Design review of the part built by this model. Coordinates are the model's own, in mm. A direction names the side the tool comes from. Give positions to 0.01 mm unless a question says otherwise; leave off trailing zeros. Loops run counter-clockwise (first coordinate to the right, second up) from the corner with the lowest first, then second, coordinate; pieces in that order, holes last. Notation, with made-up numbers: (0, -11) - (43, -11) arc R30 ccw to (43, 26) - close; hole circle Ø1 at (-15, 11). An arc over 180 degrees is marked (long way). Write each question's results on one line, items separated by ' | '.
```python
from build123d import *

# Parameters (mm, degrees)
F2_SIZE = 1


with BuildPart() as f1:
    # F0 (on Front) → F1 (revolve)
    with BuildSketch(Plane.XZ):
        Polygon((-27.5, 0), (-22, 0), (-22, 13), (-19, 13), (-19, 25), (-22, 25), (-22, 38), (-27.5, 38), (-27.5, 36), (-26, 36), (-26, 27), (-27.5, 27), (-27.5, 11), (-26, 11), (-26, 2), (-27.5, 2), align=None)
    revolve(axis=Axis((0, 0, 48.059855), (0, 0, 1)))

    # F2
    f2_edges = [f1.edges().sort_by_distance(p)[0] for p in [
        (22, 0, 38),
        (22, 0, 0),
    ]]
    chamfer(f2_edges, length=F2_SIZE)


solid = f1.part
```
Item 1: Tool access review of faces 1 (the face through (-7, -18, 25)), 2 (the face through (20.633, 15.821, 6.437)), 3 (the face through (-14.4, 18.2, 38)), 4 (the face through (7, -18, 13)): name each direction out of +Z, -Z, +X, -X, +Y, -Y from which nothing blocks a thin tool from reaching the whole face with its end or side.
Output values:
face 1: +Z | face 2: none | face 3: +Z, +X, -X, +Y, -Y | face 4: -Z
Item 2: Wall thickness on probe 1 along Z at (x, y) = (-20, -17); probe 2 along Y at (x, z) = (0, 5.5); probe 3 along Y at (x, z) = (0, 16.5): over which ranges is each line inside the solid? List them lowest first.
Output values:
probe 1: z = 0 to 2, 11 to 27, 36 to 38 | probe 2: y = -26 to -22, 22 to 26 | probe 3: y = -27.5 to -19, 19 to 27.5
Item 3: We need section B-B on y = 24. Give the boundary of the cut face in (x, z).
Output values:
outline: (-13.43, 0) - (13.43, 0) - (13.43, 2) - (10, 2) - (10, 11) - (13.43, 11) - (13.43, 27) - (10, 27) - (10, 36) - (13.43, 36) - (13.43, 38) - (-13.43, 38) - (-13.43, 36) - (-10, 36) - (-10, 27) - (-13.43, 27) - (-13.43, 11) - (-10, 11) - (-10, 2) - (-13.43, 2) - close
Item 4: Draft analysis for pull direction Y (two halves, no side actions). For faces 5 (the face through (5.961, 26.846, 36.986)), 6 (the face through (4.769, 21.477, 7.084)), 7 (the face through (-10.1, 24.3, 36)), state which applies: +Y half, -Y half, draft (parallel to the pull), parting line (faces both ways), or undercut.
Output values:
face 5: parting line | face 6: undercut | face 7: draft
Item 5: We need section A-A on z = 28.5. Give the boundary of the cut face in (x, y), then the cut area to 3 significant figures.
Output values:
outline: circle Ø52 at (0, 0); hole circle Ø44 at (0, 0) | area: 603 mm²
Item 6: We need section C-C on z = 16. Give the boundary of the cut face in (x, y).
Output values:
outline: circle Ø55 at (0, 0); hole circle Ø38 at (0, 0)
Item 7: Clearance check with flat-ended pins moving along their axes: P1, Ø2, axis at x = 1.5, z = 9.5, coming from the +Y side; P2, Ø1.5, axis at y = -8.5, z = 14, coming from the +X side; P3, Ø4, axis at x = -11, z = 28, coming from the -Y side; P4, Ø23, axis at x = 0, y = 0, coming from the +Z side. State where each tip first meets the part, or that it passes through.
Output values:
P1: stops at y = 26 | P2: stops at x = 26.39 | P3: stops at y = -25.89 | P4: passes through
